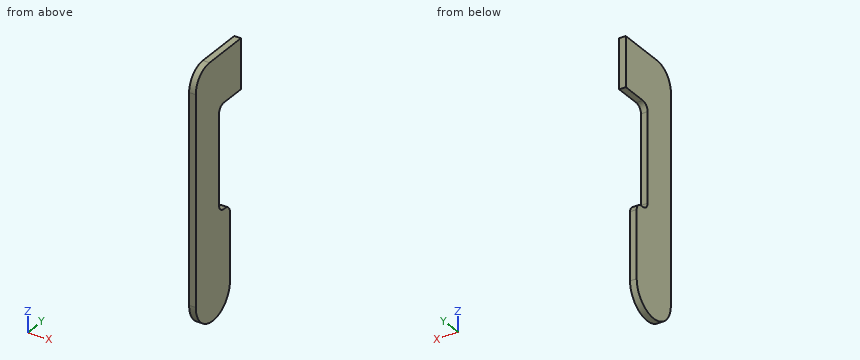
```python
from build123d import *

# Parameters (mm, degrees)
AUFSATZ_LINEAR_AUSTRAGEN1_DEPTH = 1.6


with BuildPart() as part:
    # Skizze1 → Aufsatz-Linear austragen1 (new body)
    with BuildSketch(Plane(origin=(0, 0, 0), x_dir=(0, 0, -1), z_dir=(1, 0, 0))):
        with BuildLine():
            Line((45, -12.5), (95, -12.5))
            ThreePointArc((95, -12.5), (101.25, -6.25), (95, 0))
            Line((95, 0), (78.75, 0))
            ThreePointArc((78.75, 0), (77.512563133, -0.512563133), (77, -1.75))
            Line((77, -1.75), (77, -2.25))
            ThreePointArc((77, -2.25), (76.487436867, -3.487436867), (75.25, -4))
            Line((75.25, -4), (53.75, -4))
            ThreePointArc((53.75, -4), (52.512563133, -3.487436867), (52, -2.25))
            Line((52, -2.25), (52, 4))
            Line((52, 4), (40, 4))
            Line((40, 4), (40, -4))
            Line((40, -4), (40, -7.5))
            ThreePointArc((40, -7.5), (41.464466094, -11.035533906), (45, -12.5))
        make_face()
    extrude(amount=AUFSATZ_LINEAR_AUSTRAGEN1_DEPTH)


solid = part.part
```
Geometry: final body of the model. Coordinates: model frame, mm. Give positions to 0.01 mm unless a question says otherwise; leave off trailing zeros. Loops run counter-clockwise (first coordinate to the right, second up) from the corner with the lowest first, then second, coordinate; pieces in that order, holes last. Notation, with made-up numbers: (-5, -2) -> (53, -2) arc R38 cw to (53, 36) -> close; hole circle Ø1 at (-28, 59). An arc over 180 degrees is marked (long way). Return JSON: item names as keys, results as strings.
Item 1: Section C-C, the plane z = -73.5. Output: boundary loops of the cut face in (x, y), plus the area to 3 significant figures.
Filled in:
{"outline": "(0, -12.5) -> (1.6, -12.5) -> (1.6, -4) -> (0, -4) -> close", "area": "13.6 mm^2"}
Item 2: Section A-A, the plane x = 0.7. Output: boundary loops of the cut face in (y, z), plus the area to 3 significant figures.
Filled in:
{"outline": "(-12.5, -95) arc R6.25 ccw to (0, -95) -> (0, -78.75) arc R1.75 ccw to (-1.75, -77) -> (-2.25, -77) arc R1.75 cw to (-4, -75.25) -> (-4, -53.75) arc R1.75 cw to (-2.25, -52) -> (4, -52) -> (4, -40) -> (-7.5, -40) arc R5 ccw to (-12.5, -45) -> close", "area": "692 mm^2"}
Item 3: Section B-B, the plane z = -91. Output: boundary loops of the cut face in (x, y).
Filled in:
{"outline": "(0, -12.5) -> (1.6, -12.5) -> (1.6, 0) -> (0, 0) -> close"}
Item 4: Line query: line 1 (Y direction, x = 0.95, z = -80); line 2 (Z direction, x = 0.7, y = 2); line 3 (Z direction, x = 0.35, y = -1.5). Output: solid intervals per line, ascending.
Filled in:
{"line 1": "-12.5 to 0", "line 2": "-52 to -40", "line 3": "-99.06 to -77.02, -52 to -40"}
Item 5: Pin query (flat end, axial travel): P1, Ø0.8, axis at x = 1, z = -62.5, coming from the +Y side; P2, Ø0.5, axis at x = 0.5, y = 2, coming from the -Z side; P3, Ø6, axis at y = -8.5, z = -77.5, coming from the -X side. Return the tip coordinate at first contact, or that it passes through.
Filled in:
{"P1": "y = -4", "P2": "z = -52", "P3": "x = 0"}
